Could you check a few things on this model? Use its own coordinates, in mm. A direction names the side the tool comes from. Round coordinates to 2 decimals unless told otherwise and drop trailing zeros. Loops run counter-clockwise (first coordinate to the right, second up) from the corner with the lowest first, then second, coordinate; pieces in that order, holes last. Notation, with made-up numbers: (-20, 12) -> (18, 12) arc R24 ccw to (18, 32) -> close; hole circle Ø7 at (-25, 57). An arc over 180 degrees is marked (long way). One line per item, written item: value.
```python
from build123d import *

# Parameters (mm, degrees)
F0_W        = 75.0949196517
F0_H        = 14.2217068933
F0_W_2      = 22.86
F0_H_2      = 3.556
F1_DEPTH    = 101.6
F2_T1_DEPTH = 165.9870757085
F3_R        = 6.5531023684
F4_SIZE2    = 6.0344471764
F4_SIZE     = 38.1
F4_2_SIZE2  = 6.0344471764
F4_2_SIZE   = 38.1
F5_T1_DEPTH = 234.6078157438
F6_T1_DEPTH = 118.09821105


# Not quite as in the source:
# - a fillet or chamfer that OpenCascade refuses, or shapes differently, is made with other operations: its cross-section is extruded or revolved along the edge and cut away or added


with BuildPart() as f1:
    # F0 (on Top) → F1 (new body)
    with BuildSketch(Plane.XY):
        with Locations((7.2930697352, -0.4826590884)):
            Rectangle(F0_W, F0_H)
        Rectangle(F0_W_2, F0_H_2, mode=Mode.SUBTRACT)
    extrude(amount=F1_DEPTH)

    # F2: fillet of radius 12.8774151417 on 1 edges, made by hand

    # F2_s2 → F2_t1 (cut)
    with BuildSketch(Plane.XY.offset(-32.1935378542)):
        with BuildLine():
            add(Edge.make_bspline(
                [(-17.376974949, 6.6281943582), (-30.2543900907, 6.6281943582), (-30.2543900907, -6.2492207835)],
                knots=[0, 0, 0, 1, 1, 1], degree=2, weights=[1, 1, 1]))
            Line((-30.2543900907, -6.2492207835), (-30.2543900907, 6.6281943582))
            Line((-30.2543900907, 6.6281943582), (-17.376974949, 6.6281943582))
        make_face()
    extrude(amount=F2_T1_DEPTH, mode=Mode.SUBTRACT)

    # F3
    f3_edges = [f1.edges().sort_by_distance(p)[0] for p in [
        (-30.25439, -7.593513, 50.8),
    ]]
    fillet(f3_edges, radius=F3_R)

    # F4
    f4_edges = [f1.edges().sort_by_distance(p)[0] for p in [
        (44.84053, 6.628194, 50.8),
    ]]
    f4_side = f1.faces().sort_by_distance((13.731777, 6.628194, 50.8))[0]
    chamfer(f4_edges, length=F4_SIZE, length2=F4_SIZE2, reference=f4_side)

    # F4#2
    f4_2_edges = [f1.edges().sort_by_distance(p)[0] for p in [
        (44.84053, -7.593513, 50.8),
    ]]
    f4_2_side = f1.faces().sort_by_distance((11.322316, -7.593513, 50.8))[0]
    chamfer(f4_2_edges, length=F4_2_SIZE, length2=F4_2_SIZE2, reference=f4_2_side)

    # F5: fillet of radius 171.7049577379 on 1 edges, made by hand

    # F5_s2 → F5_t1 (cut)
    with BuildSketch(Plane.XY.offset(-66.5039078719)):
        with BuildLine():
            ThreePointArc((44.840529561, -1.5590653587), (31.8279082353, 2.1157050987), (18.5664757974, 4.7551484822))
            Line((18.5664757974, 4.7551484822), (44.840529561, 0.5937471818))
            Line((44.840529561, 0.5937471818), (44.840529561, -1.5590653587))
        make_face()
    extrude(amount=F5_T1_DEPTH, mode=Mode.SUBTRACT)

    # F6: fillet of radius 0.7744916247 on 1 edges, made by hand

    # F6_s2 → F6_t1 (cut)
    with BuildSketch(Plane.XY.offset(-8.249105525)):
        with BuildLine():
            ThreePointArc((41.5888697855, -2.0740776724), (42.240352702, -1.3626428472), (41.6931850181, -0.5681763427))
            ThreePointArc((41.6931850181, -0.5681763427), (43.2692375752, -1.0560603886), (44.840529561, -1.5590653587))
            Line((44.840529561, -1.5590653587), (41.5888697855, -2.0740776724))
        make_face()
    extrude(amount=F6_T1_DEPTH, mode=Mode.SUBTRACT)


solid = f1.part
```
Item 1: If we section it at A-A on x = 1: List the corners of the cut face in (y, z) for me, plus the area to 3 significant figures.
Output:
outline: (-7.59, 0) -> (-1.78, 0) -> (-1.78, 101.6) -> (-7.59, 101.6) -> close; (1.78, 0) -> (6.63, 0) -> (6.63, 101.6) -> (1.78, 101.6) -> close
area: 1,080 mm²
Item 2: For faces 5 (the face through (0, 1.778, 50)), 6 (the face through (-8, -7.594, 50)), which set-ups out of +Z, -Z, +X, -X, +Y, -Y let a thin tool reach every point of the face, with its end or its side?
Output:
face 5: +Z, -Z
face 6: +Z, -Z, +X, -X, -Y
Item 3: If we section it at C-C on x = 28: List the corners of the cut face in (y, z) for me, plus the area to 3 significant figures.
Output:
outline: (-4.23, 0) -> (2.99, 0) -> (2.99, 101.6) -> (-4.23, 101.6) -> close
area: 733 mm²
Item 4: I need wall thicknesses on line 1 (Y direction, x = -9.5, z = 29); line 2 (Y direction, x = -18, z = 14); line 3 (Y direction, x = 31, z = 6). Which ranges of each line are inside material? Lowest first, please. Write a range as from..to.
Output:
line 1: y = -7.59..-1.78, 1.78..6.63
line 2: y = -7.59..6.62
line 3: y = -3.75..2.31
Item 5: Will these pins go through, and if not, where does the flat tip stop? pin 1 Ø1.5 at (x, y) = (26.5, 4) entering from +Z; pin 2 Ø10 at (x, z) = (17, 28) entering from +Y.
Output:
pin 1: stops at z = 101.6
pin 2: stops at y = 5.8
Item 6: If we section it at B-B on x = 15: List the corners of the cut face in (y, z) for me, plus the area to 3 significant figures.
Output:
outline: (-6.29, 0) -> (5.32, 0) -> (5.32, 101.6) -> (-6.29, 101.6) -> close
area: 1,180 mm²
Item 7: If we mould it in two halves opening along X, with no side actions, what happens to faces 1 (the face through (30.384, 2.456, 50.089)), 2 (the face through (11.43, 0, 50)), 3 (the face through (-2, -2, 0)), 4 (the face through (0, -1.778, 50))? For each: released by +X, released by -X, zero draft, split by the parting line, or undercut.
Output:
face 1: released by +X
face 2: undercut
face 3: zero draft
face 4: undercut
